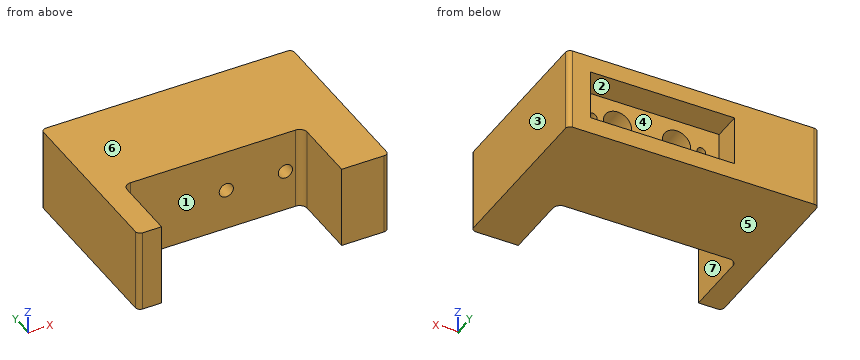
Autodesk Inventor part; units mm, degrees
ref_plane "YZ Plane" through (0, 0, 0) normal (1, 0, 0) x (0, 1, 0)
ref_plane "XZ Plane" through (0, 0, 0) normal (0, 1, 0) x (-1, 0, 0)
ref_plane "XY Plane" through (0, 0, 0) normal (0, 0, 1) x (1, 0, 0)
sketch "Sketch1" plane through (0, 0, 0) normal (0, 1, 0) x (-1, 0, 0)
  line L0 (0, 0) -> (60, 0) construction
  line L1 (60, 0) -> (60, -20) construction
  line L2 (60, -20) -> (0, -20) construction
  line L3 (0, -20) -> (0, 0) construction
  line L4 (60.5, 0.5) -> (-0.5, 0.5)
  line L5 (-0.5, 0.5) -> (-0.5, -20.5)
  line L6 (-0.5, -20.5) -> (60.5, -20.5)
  line L7 (60.5, -20.5) -> (60.5, 0.5)
  circle A0 centre (53, -10) radius 1.8
  circle A1 centre (7, -10) radius 1.8
  line L8 (53, -10) -> (7, -10) construction
  point P0 (30, -10)
  point P1 (30, -20)
  point P2 (7, -10)
  point P3 (0, -10)
  dimension "d0" = 20
  dimension "d1" = 60
  dimension "d2" = 0.5
  dimension "d3" = 0.5
  dimension "d4" = 0.5
  dimension "d5" = 0.5
  dimension "d6" = 3.6
  dimension "d7" = 46
sketch "Sketch2" plane through (0, 0, 0) normal (0, 1, 0) x (-1, 0, 0)
  line L0 (-10, 7.5) -> (96.2, 7.5)
  line L1 (96.2, 7.5) -> (96.2, -27.5)
  line L2 (96.2, -27.5) -> (-10, -27.5)
  line L3 (-10, -27.5) -> (-10, 7.5)
  line L4 (60.5, -20.5) -> (60.5, 0.5) construction
  line L5 (-0.5, 0.5) -> (-0.5, -20.5) construction
  line L6 (-0.5, -20.5) -> (60.5, -20.5) construction
  point P0 (0, 0)
  point P1 (60.5, -10)
  point P2 (96.2, -10)
  point P3 (30, -20.5)
  point P4 (43.1, -27.5)
  dimension "d9" = 106.2
  dimension "d10" = 35
  dimension "d43" = 10
extrude "Extrusion1" add sketch "Sketch2" along normal blind 10 and the other way blind 35.4
extrude "Extrusion2" cut sketch "Sketch1" along normal blind 10 and the other way blind 2
extrude "Extrusion3" cut sketch "Sketch1" along normal blind 10 and the other way blind 30.4 contours A0 | A1
sketch "Sketch3" plane through (10, 10, -27.5) normal (0, 0, -1) x (-1, 0, 0)
  line L0 (106.2, -45.4) -> (0, -45.4)
  line L1 (0, -45.4) -> (0, -75.4)
  line L2 (0, -75.4) -> (20, -75.4)
  line L3 (20, -75.4) -> (20, -48.575)
  line L4 (23.175, -45.4) -> (93.025, -45.4)
  line L5 (96.2, -48.575) -> (96.2, -75.4)
  line L6 (96.2, -75.4) -> (106.2, -75.4)
  line L7 (106.2, -75.4) -> (106.2, -45.4)
  arc A0 (23.175, -45.4) -> (20, -48.575) centre (23.175, -48.575) ccw
  arc A1 (96.2, -48.575) -> (93.025, -45.4) centre (93.025, -48.575) ccw
  point P0 (10, -10)
  point P1 (20, -45.4)
  point P2 (96.2, -45.4)
  point P3 (53.1, -45.4)
  point P4 (93.025, -45.4)
  dimension "d23" = 76.2
  dimension "d24" = 3.175
  dimension "d25" = 20
  dimension "d26" = 30
extrude "Extrusion4" add sketch "Sketch3" against normal up to surface (35 mm away)
sketch "Sketch4" plane through (0, -2, 0) normal (0, 1, 0) x (1, 0, 0)
  circle A0 centre (-42.5, 10) radius 3
  circle A1 centre (-17.5, 10) radius 3
  line L0 (-60.5, 20.5) -> (0.5, 20.5) construction
  line L1 (-60.5, -0.5) -> (-60.5, 20.5) construction
  line L2 (-42.5, 10) -> (-17.5, 10) construction
  point P0 (0, 0)
  point P1 (-30, 20.5)
  point P2 (-30, 10)
  point P3 (-60.5, 10)
  dimension "d29" = 6
  dimension "d30" = 25
extrude "Extrusion5" cut sketch "Sketch4" against normal up to surface (33.4 mm away)
sketch "Sketch5" plane through (0, -2, 0) normal (0, 1, 0) x (1, 0, 0)
  circle A0 centre (-42.5, 10) radius 3 construction
  circle A1 centre (-17.5, 10) radius 3 construction
  circle A2 centre (-17.5, 10) radius 6
  circle A3 centre (-42.5, 10) radius 6
  point P0 (0, 0)
  dimension "d34" = 12
extrude "Extrusion6" cut sketch "Sketch5" against normal blind 10
fillet "Fillet1" radius 2 2 edges at (-96.2, 10, -10) (10, 10, -10)
fillet "Fillet2" radius 2 2 edges at (-96.2, -65.4, -10) (10, -65.4, -10)
properties part number "BK12_Spacer"
The listing builds one solid part. Answer for the finished solid, in the listing's coordinates (mm). Face numbers are marked on the shaded views. A direction names the side the tool comes from. Give positions to 0.01 mm unless a question says otherwise; leave off trailing zeros. Loops run counter-clockwise (first coordinate to the right, second up) from the corner with the lowest first, then second, coordinate; pieces in that order, holes last. Notation, with made-up numbers: (-32, -4) - (-21, -4) arc R21 ccw to (-21, 35) - close; hole circle Ø8 at (22.5, 86.5). An arc over 180 degrees is marked (long way). Answer as CSV lines item,"result". Start each with the question number.
Item 1: A cutting plane is placed at C-C on y = -17.5. Determine the outline of the cut face in (x, z).
Item 2: A cutting plane is placed at D-D on x = -17.5. Determine the outline of the cut face in (y, z).
Item 3: For the marked faces 1, 2 and 3, determine the directions among +Z, -Z, +X, -X, +Y, -Y from which every point of the face is accessible in a straight line to the end or side of a thin tool.
Item 4: A cutting plane is placed at B-B on x = -53. Determine the outline of the cut face in (y, z).
Item 5: Each of these flat-tipped pins is pushed along its axis until it touches: pin 1 (2 mm diameter, centred on x = -32.5, z = -5, fed in from -Y); pin 2 (6 mm diameter, centred on x = -41.5, z = -7.5, fed in from +Y); pin 3 (1.8 mm diameter, centred on x = -53, z = -11, fed in from +Y); pin 4 (5 mm diameter, centred on x = -42.5, z = -10, fed in from +Y). Where does it stop, or does it pass through?
Item 6: Find the intervals of material crossed by line 1 (X direction, y = -45.5, z = -1.5); line 2 (X direction, y = 6.5, z = -10); line 3 (Y direction, x = -57.5, z = 1.5), in increasing order. Write a range as from..to.
Item 7: A cutting plane is placed at A-A on y = -57. Determine the outline of the cut face in (x, z), then the cut area to 3 significant figures.
Item 8: The mould has two halves that part along Z. Classify the marked faces 4, 5, 6 and 7: +Z half, -Z half, draft (parallel to the pull), parting line (faces both ways), or undercut.
Found:
1,outline,"(-96.2, -27.5) - (10, -27.5) - (10, 7.5) - (-96.2, 7.5) - close; hole circle Ø3.6 at (-53, -10); hole circle Ø6 at (-42.5, -10); hole circle Ø6 at (-17.5, -10); hole circle Ø3.6 at (-7, -10)"
2,outline,"(-35.4, -27.5) - (10, -27.5) - (10, -20.5) - (-2, -20.5) - (-2, -16) - (-12, -16) - (-12, -13) - (-35.4, -13) - close; (-35.4, -7) - (-12, -7) - (-12, -4) - (-2, -4) - (-2, 0.5) - (10, 0.5) - (10, 7.5) - (-35.4, 7.5) - close"
3,face 1,"+Z, -Z, -Y"
3,face 2,"+Y"
3,face 3,"+Z, -Z, +X, +Y, -Y"
4,outline,"(-35.4, -27.5) - (10, -27.5) - (10, -20.5) - (-2, -20.5) - (-2, -11.8) - (-30.4, -11.8) - (-30.4, -8.2) - (-2, -8.2) - (-2, 0.5) - (10, 0.5) - (10, 7.5) - (-35.4, 7.5) - close"
5,pin 1,"stops at y = -35.4"
5,pin 2,"stops at y = -12"
5,pin 3,"stops at y = -2"
5,pin 4,"passes through"
6,line 1,"x = -96.2..-86.2, -10..10"
6,line 2,"x = -96.2..-60.5, 0.5..10"
6,line 3,"y = -35.4..10"
7,outline,"(-96.2, -27.5) - (-86.2, -27.5) - (-86.2, 7.5) - (-96.2, 7.5) - close; (-10, -27.5) - (10, -27.5) - (10, 7.5) - (-10, 7.5) - close"
7,area,"1,050 mm^2"
8,face 4,"undercut"
8,face 5,"-Z half"
8,face 6,"+Z half"
8,face 7,"draft"
